from build123d import *

# Parameters (mm, degrees)
BOSS_EXTRUDE1_DEPTH     = 100
SKETCH1_3_R             = 12.5
BOSS_EXTRUDE2_DEPTH     = 20
BOSS_EXTRUDE3_START     = -100
SKETCH1_4_W             = 20
SKETCH1_4_H             = 12
BOSS_EXTRUDE3_DEPTH     = 70
BOSS_EXTRUDE4_START     = -55
SKETCH2_R               = 12.5
BOSS_EXTRUDE4_DEPTH     = 20
BOSS_EXTRUDE5_START     = -125
SKETCH2_3_R             = 12.5
BOSS_EXTRUDE5_DEPTH     = 20
CUT_EXTRUDE1_DEPTH      = 209.315712821
CUT_EXTRUDE1_DEPTH_BACK = 209.315712821
SKETCH4_W               = 20
SKETCH4_H               = 20


with BuildPart() as part:
    # Sketch1 → Boss-Extrude1 (new body)
    with BuildSketch(Plane.XY):
        Polygon((105, 20), (125, 20), (160, 20), (160, 0), (0, 0), (0, 20), (35, 20), (55, 20), align=None)
    extrude(amount=-BOSS_EXTRUDE1_DEPTH)

    # Sketch1<3> → Boss-Extrude2 (add)
    with BuildSketch(Plane.XY):
        with BuildLine():
            Line((105, 0), (55, 0))
            Line((55, 0), (55, -27))
            ThreePointArc((55, -27), (80, -52), (105, -27))
            Line((105, -27), (105, 0))
        make_face()
        with Locations((80, -27)):
            Circle(SKETCH1_3_R, mode=Mode.SUBTRACT)
    extrude(amount=-BOSS_EXTRUDE2_DEPTH)

    # Sketch1<4> → Boss-Extrude3 (add)
    with BuildSketch(Plane.XY.offset(BOSS_EXTRUDE3_START)):
        with Locations((80, 26)):
            Rectangle(SKETCH1_4_W, SKETCH1_4_H)
    extrude(amount=BOSS_EXTRUDE3_DEPTH)

    # Sketch2 → Boss-Extrude4 (add)
    with BuildSketch(Plane.ZY.offset(BOSS_EXTRUDE4_START)):
        with BuildLine():
            Line((0, 20), (-43.758397368, 95.791767499))
            ThreePointArc((-43.758397368, 95.791767499), (-79.070979034, 104.228606226), (-85.569779349, 68.508524114))
            Line((-85.569779349, 68.508524114), (-50, 20))
            Line((-50, 20), (0, 20))
        make_face()
        with Locations((-65.409032463, 83.291767499)):
            Circle(SKETCH2_R, mode=Mode.SUBTRACT)
    extrude(amount=BOSS_EXTRUDE4_DEPTH)

    # Sketch2<3> → Boss-Extrude5 (add)
    with BuildSketch(Plane.ZY.offset(BOSS_EXTRUDE5_START)):
        with BuildLine():
            Line((0, 20), (-43.758397368, 95.791767499))
            ThreePointArc((-43.758397368, 95.791767499), (-79.070979034, 104.228606226), (-85.569779349, 68.508524114))
            Line((-85.569779349, 68.508524114), (-50, 20))
            Line((-50, 20), (0, 20))
        make_face()
        with Locations((-65.409032463, 83.291767499)):
            Circle(SKETCH2_3_R, mode=Mode.SUBTRACT)
    extrude(amount=BOSS_EXTRUDE5_DEPTH)

    # Sketch4 → Cut-Extrude1 (cut, two sides: drawn at the far end of the back side and taken through both)
    with BuildSketch(Plane(origin=(0, 20, 0), x_dir=(1, 0, 0), z_dir=(0, 1, 0)).offset(-CUT_EXTRUDE1_DEPTH_BACK)):
        Polygon((0, 100), (0, 80), (35, 100), align=None)
        Polygon((0, 0), (35, 0), (0, 40), align=None)
        Polygon((160, 40), (125, 0), (160, 0), align=None)
        Polygon((125, 100), (160, 80), (160, 100), align=None)
        with Locations((150, 60)):
            Rectangle(SKETCH4_W, SKETCH4_H)
        with Locations((10, 60)):
            Rectangle(SKETCH4_W, SKETCH4_H)
    extrude(amount=CUT_EXTRUDE1_DEPTH + CUT_EXTRUDE1_DEPTH_BACK, mode=Mode.SUBTRACT)


solid = part.part
Design review of the part built by this model. Coordinates are the model's own, in mm. A direction names the side the tool comes from. Give positions to 0.01 mm unless a question says otherwise; leave off trailing zeros. Order: outer loops, then holes, each group sorted by start corner. A loop starts at its lowest first (then second) coordinate and runs counter-clockwise, first axis right, second up.
1. To check wall thickness, follow L1, parallel to X at y = 21.5, z = -35.5; L2, parallel to X at y = 74, z = -44.5; L3, parallel to Y at x = 49, z = -66. State the ranges of each line that lie inside material, in increasing order.
Solution:
L1: x = 35 to 55, 70 to 90, 105 to 125
L2: x = 35 to 55, 105 to 125
L3: y = 0 to 20, 41.82 to 70.81, 95.78 to 108.28
2. Add section D-D, the plane x = 96. State the section outline as (y, z) points, then the cut area to 3 significant figures.
Solution:
outline: (-46.21, -20) - (0, -20) - (0, -100) - (20, -100) - (20, 0) - (-46.21, 0) - close
area: 2,920 mm2
3. For pin 1 Ø25 at (x, y) = (87, -14) entering from -Z; pin 2 Ø6 at (x, y) = (7, 12.5) entering from -Z; pin 3 Ø3.5 at (x, y) = (75.5, 27.5) entering from +Z, all flat-tipped, find the tip position at first contact; note any pin that passes through.
Solution:
pin 1: stops at z = -20
pin 2: stops at z = -85.71
pin 3: stops at z = -30
4. Add section C-C, the plane z = -34. State the section outline as (x, y) points, then the cut area to 3 significant figures.
Solution:
outline: (5.25, 0) - (154.75, 0) - (154.75, 20) - (125, 20) - (125, 78.89) - (105, 78.89) - (105, 20) - (90, 20) - (90, 32) - (70, 32) - (70, 20) - (55, 20) - (55, 78.89) - (35, 78.89) - (35, 20) - (5.25, 20) - close
area: 5,590 mm2
5. Mouldability with a two-part tool opening along Y and no side actions: class faces 5 (the flat face through (45.14, 57.365, -21.573)), 6 (the cylindrical face through (79.45, -51.994, -9.86)), 7 (the flat face through (160, 10, -75)), 8 (the cylindrical face through (91.547, -31.788, -9.86)) as +Y half, -Y half, draft (parallel to the pull), parting line (faces both ways), or undercut.
Solution:
face 5: +Y half
face 6: -Y half
face 7: draft
face 8: undercut
6. Tool access review of faces 1 (the flat face through (55, 65, -46)), 2 (the flat face through (35, 65, -46)), 3 (the flat face through (10, 10, -50)), 4 (the flat face through (150, 10, -50)): name each direction out of +Z, -Z, +X, -X, +Y, -Y from which nothing blocks a thin tool from reaching the whole face with its end or side.
Solution:
face 1: +Z, -Z, +Y
face 2: +Z, -Z, -X, +Y
face 3: -X, +Y, -Y
face 4: +X, +Y, -Y
7. Add section A-A, the plane x = 80. State the section outline as (y, z) points.
Solution:
outline: (-52, -20) - (-39.5, -20) - (-39.5, 0) - (-52, 0) - close; (-14.5, -20) - (0, -20) - (0, -100) - (32, -100) - (32, -30) - (20, -30) - (20, 0) - (-14.5, 0) - close
8. Add section B-B, the plane z = -75. State the section outline as (x, y) points, then the cut area to 3 significant figures.
Solution:
outline: (0, 0) - (160, 0) - (160, 20) - (90, 20) - (90, 32) - (70, 32) - (70, 20) - (0, 20) - close; (35, 54.09) - (55, 54.09) - (55, 75.28) - (35, 75.28) - close; (35, 91.31) - (55, 91.31) - (55, 106.38) - (35, 106.38) - close; (105, 54.09) - (125, 54.09) - (125, 75.28) - (105, 75.28) - close; (105, 91.31) - (125, 91.31) - (125, 106.38) - (105, 106.38) - close
area: 4,890 mm2
